Here's how the part is built. I have some questions about the finished solid (model axes, mm). A direction names the side the tool comes from. Give positions to 0.01 mm unless a question says otherwise; leave off trailing zeros. Loops run counter-clockwise (first coordinate to the right, second up) from the corner with the lowest first, then second, coordinate; pieces in that order, holes last.
Q1. I need wall thicknesses on probe 1 along X at (y, z) = (-7, 2.15) (3 decimals); probe 2 along Y at (x, z) = (52, 2.4) (3 decimals); probe 3 along X at (y, z) = (48, 2.1). Which ranges of each line are inside material? Lowest first, please.
Q2. Suppose I cut it at C-C (x = 69). List the corners of the cut face in (y, z) for me (3 decimals), and give its area (3 significant figures).
Q3. Thinking about a two-plate mould opening in X: for faces 1 (the face through (37, -4, 0)), 2 (the face through (28, -36.675, 1)), 3 (the face through (9, -17.625, 1)), 4 (the face through (-13.852, -62.211, 1.479)), which applies, pulls with the +X half, pulls with the -X half, needs draft (parallel to the pull), parting line crosses it, or undercut?
Q4. Suppose I cut it at D-D (z = 1.4). Count the separate pieces of the cut face and the enclosed holes in it, and give its area (3 significant figures).
Q5. Suppose I cut it at B-B (y = -1). List the corners of the cut face in (x, z) for me (3 decimals).
Q6. For faces 5 (the face through (28.817, 39, 1)), 6 (the face through (-15.278, -4, 1)), 7 (the face through (2.525, -44, 1)), which set-ups out of +Z, -Z, +X, -X, +Y, -Y let a thin tool reach every point of the face, with its end or its side?
Q7. I'm going to push flat-ended pins straight in: P1, Ø1, axis at x = 35, z = 1, coming from the +Y side; P2, Ø5, axis at x = 54, y = 35.5, coming from the -Z side. Where does each tip first touch, or does it pass through?
Q8. Suppose I cut it at A-A (y = 31). List the corners of the cut face in (x, z) for me, and give its area (3 significant figures).
```python
from build123d import *

# Parameters (mm, degrees)
SKETCH_R     = 1.7
PAD_DEPTH    = 3
POCKET_DEPTH = 10


with BuildPart() as part:
    # Sketch → Pad (new body)
    with BuildSketch(Plane.XY):
        with BuildLine():
            Line((-15.278, 48.916), (-15.278, -58.715))
            ThreePointArc((-15.278, -58.715), (-13.813534, -62.250534), (-10.278, -63.715))
            Line((-10.278, -63.715), (85.447, -63.715))
            ThreePointArc((85.447, -63.715), (88.982534, -62.250534), (90.447, -58.715))
            Line((90.447, -58.715), (90.447, 48.916))
            ThreePointArc((90.447, 48.916), (88.982534, 52.451534), (85.447, 53.916))
            Line((85.447, 53.916), (47.31676, 53.916))
            Line((47.31676, 22.916), (47.31676, 53.916))
            Line((28.81676, 22.916), (47.31676, 22.916))
            Line((28.81676, 53.916), (28.81676, 22.916))
            Line((28.81676, 53.916), (-10.278, 53.916))
            ThreePointArc((-10.278, 53.916), (-13.813534, 52.451534), (-15.278, 48.916))
        make_face()
        with Locations((-10.278, -58.715)):
            Circle(SKETCH_R, mode=Mode.SUBTRACT)
        with Locations((-10.278, 48.916)):
            Circle(SKETCH_R, mode=Mode.SUBTRACT)
        with Locations((85.447, 48.916)):
            Circle(SKETCH_R, mode=Mode.SUBTRACT)
        with Locations((85.447, -58.715)):
            Circle(SKETCH_R, mode=Mode.SUBTRACT)
    extrude(amount=PAD_DEPTH)

    # Sketch001 → Pocket (cut)
    with BuildSketch(Plane(origin=(0, 23, 0), x_dir=(1, 0, 0), z_dir=(0, 0, 1))):
        with BuildLine():
            ThreePointArc((73.175, -73.675), (73.528553, -73.528553), (73.675, -73.175))
            Line((73.675, -60.175), (73.675, -73.175))
            ThreePointArc((73.675, -60.175), (73.528553, -59.821447), (73.175, -59.675))
            Line((60.175, -59.675), (73.175, -59.675))
            ThreePointArc((60.175, -59.675), (59.821447, -59.821447), (59.675, -60.175))
            Line((59.675, -60.175), (59.675, -73.175))
            ThreePointArc((59.675, -73.175), (59.821447, -73.528553), (60.175, -73.675))
            Line((60.175, -73.675), (73.175, -73.675))
        make_face()
        with BuildLine():
            Line((3.025, -2.525), (16.025, -2.525))
            ThreePointArc((16.525, -3.025), (16.378553, -2.671447), (16.025, -2.525))
            Line((16.525, -3.025), (16.525, -16.025))
            ThreePointArc((16.025, -16.525), (16.378553, -16.378553), (16.525, -16.025))
            Line((3.025, -16.525), (16.025, -16.525))
            ThreePointArc((2.525, -16.025), (2.671447, -16.378553), (3.025, -16.525))
            Line((2.525, -3.025), (2.525, -16.025))
            ThreePointArc((3.025, -2.525), (2.671447, -2.671447), (2.525, -3.025))
        make_face()
        with BuildLine():
            Line((22.075, -2.525), (35.075, -2.525))
            ThreePointArc((35.575, -3.025), (35.428553, -2.671447), (35.075, -2.525))
            Line((35.575, -3.025), (35.575, -16.025))
            ThreePointArc((35.075, -16.525), (35.428553, -16.378553), (35.575, -16.025))
            Line((22.075, -16.525), (35.075, -16.525))
            ThreePointArc((21.575, -16.025), (21.721447, -16.378553), (22.075, -16.525))
            Line((21.575, -3.025), (21.575, -16.025))
            ThreePointArc((22.075, -2.525), (21.721447, -2.671447), (21.575, -3.025))
        make_face()
        with BuildLine():
            Line((41.125, -2.525), (54.125, -2.525))
            ThreePointArc((54.625, -3.025), (54.478553, -2.671447), (54.125, -2.525))
            Line((54.625, -3.025), (54.625, -16.025))
            ThreePointArc((54.125, -16.525), (54.478553, -16.378553), (54.625, -16.025))
            Line((41.125, -16.525), (54.125, -16.525))
            ThreePointArc((40.625, -16.025), (40.771447, -16.378553), (41.125, -16.525))
            Line((40.625, -3.025), (40.625, -16.025))
            ThreePointArc((41.125, -2.525), (40.771447, -2.671447), (40.625, -3.025))
        make_face()
        with BuildLine():
            Line((60.175, -2.525), (73.175, -2.525))
            ThreePointArc((73.675, -3.025), (73.528553, -2.671447), (73.175, -2.525))
            Line((73.675, -3.025), (73.675, -16.025))
            ThreePointArc((73.175, -16.525), (73.528553, -16.378553), (73.675, -16.025))
            Line((60.175, -16.525), (73.175, -16.525))
            ThreePointArc((59.675, -16.025), (59.821447, -16.378553), (60.175, -16.525))
            Line((59.675, -3.025), (59.675, -16.025))
            ThreePointArc((60.175, -2.525), (59.821447, -2.671447), (59.675, -3.025))
        make_face()
        with BuildLine():
            Line((3.025, -21.575), (16.025, -21.575))
            ThreePointArc((16.525, -22.075), (16.378553, -21.721447), (16.025, -21.575))
            Line((16.525, -22.075), (16.525, -35.075))
            ThreePointArc((16.025, -35.575), (16.378553, -35.428553), (16.525, -35.075))
            Line((3.025, -35.575), (16.025, -35.575))
            ThreePointArc((2.525, -35.075), (2.671447, -35.428553), (3.025, -35.575))
            Line((2.525, -22.075), (2.525, -35.075))
            ThreePointArc((3.025, -21.575), (2.671447, -21.721447), (2.525, -22.075))
        make_face()
        with BuildLine():
            Line((22.075, -21.575), (35.075, -21.575))
            ThreePointArc((35.575, -22.075), (35.428553, -21.721447), (35.075, -21.575))
            Line((35.575, -22.075), (35.575, -35.075))
            ThreePointArc((35.075, -35.575), (35.428553, -35.428553), (35.575, -35.075))
            Line((22.075, -35.575), (35.075, -35.575))
            ThreePointArc((21.575, -35.075), (21.721447, -35.428553), (22.075, -35.575))
            Line((21.575, -22.075), (21.575, -35.075))
            ThreePointArc((22.075, -21.575), (21.721447, -21.721447), (21.575, -22.075))
        make_face()
        with BuildLine():
            Line((41.125, -21.575), (54.125, -21.575))
            ThreePointArc((54.625, -22.075), (54.478553, -21.721447), (54.125, -21.575))
            Line((54.625, -22.075), (54.625, -35.075))
            ThreePointArc((54.125, -35.575), (54.478553, -35.428553), (54.625, -35.075))
            Line((41.125, -35.575), (54.125, -35.575))
            ThreePointArc((40.625, -35.075), (40.771447, -35.428553), (41.125, -35.575))
            Line((40.625, -22.075), (40.625, -35.075))
            ThreePointArc((41.125, -21.575), (40.771447, -21.721447), (40.625, -22.075))
        make_face()
        with BuildLine():
            Line((60.175, -21.575), (73.175, -21.575))
            ThreePointArc((73.675, -22.075), (73.528553, -21.721447), (73.175, -21.575))
            Line((73.675, -22.075), (73.675, -35.075))
            ThreePointArc((73.175, -35.575), (73.528553, -35.428553), (73.675, -35.075))
            Line((60.175, -35.575), (73.175, -35.575))
            ThreePointArc((59.675, -35.075), (59.821447, -35.428553), (60.175, -35.575))
            Line((59.675, -22.075), (59.675, -35.075))
            ThreePointArc((60.175, -21.575), (59.821447, -21.721447), (59.675, -22.075))
        make_face()
        with BuildLine():
            Line((3.025, -40.625), (16.025, -40.625))
            ThreePointArc((16.525, -41.125), (16.378553, -40.771447), (16.025, -40.625))
            Line((16.525, -41.125), (16.525, -54.125))
            ThreePointArc((16.025, -54.625), (16.378553, -54.478553), (16.525, -54.125))
            Line((3.025, -54.625), (16.025, -54.625))
            ThreePointArc((2.525, -54.125), (2.671447, -54.478553), (3.025, -54.625))
            Line((2.525, -41.125), (2.525, -54.125))
            ThreePointArc((3.025, -40.625), (2.671447, -40.771447), (2.525, -41.125))
        make_face()
        with BuildLine():
            Line((22.075, -40.625), (35.075, -40.625))
            ThreePointArc((35.575, -41.125), (35.428553, -40.771447), (35.075, -40.625))
            Line((35.575, -41.125), (35.575, -54.125))
            ThreePointArc((35.075, -54.625), (35.428553, -54.478553), (35.575, -54.125))
            Line((22.075, -54.625), (35.075, -54.625))
            ThreePointArc((21.575, -54.125), (21.721447, -54.478553), (22.075, -54.625))
            Line((21.575, -41.125), (21.575, -54.125))
            ThreePointArc((22.075, -40.625), (21.721447, -40.771447), (21.575, -41.125))
        make_face()
        with BuildLine():
            Line((41.125, -40.625), (54.125, -40.625))
            ThreePointArc((54.625, -41.125), (54.478553, -40.771447), (54.125, -40.625))
            Line((54.625, -41.125), (54.625, -54.125))
            ThreePointArc((54.125, -54.625), (54.478553, -54.478553), (54.625, -54.125))
            Line((41.125, -54.625), (54.125, -54.625))
            ThreePointArc((40.625, -54.125), (40.771447, -54.478553), (41.125, -54.625))
            Line((40.625, -41.125), (40.625, -54.125))
            ThreePointArc((41.125, -40.625), (40.771447, -40.771447), (40.625, -41.125))
        make_face()
        with BuildLine():
            Line((60.175, -40.625), (73.175, -40.625))
            ThreePointArc((73.675, -41.125), (73.528553, -40.771447), (73.175, -40.625))
            Line((73.675, -41.125), (73.675, -54.125))
            ThreePointArc((73.175, -54.625), (73.528553, -54.478553), (73.675, -54.125))
            Line((60.175, -54.625), (73.175, -54.625))
            ThreePointArc((59.675, -54.125), (59.821447, -54.478553), (60.175, -54.625))
            Line((59.675, -41.125), (59.675, -54.125))
            ThreePointArc((60.175, -40.625), (59.821447, -40.771447), (59.675, -41.125))
        make_face()
        with BuildLine():
            Line((3.025, -59.675), (16.025, -59.675))
            ThreePointArc((16.525, -60.175), (16.378553, -59.821447), (16.025, -59.675))
            Line((16.525, -60.175), (16.525, -73.175))
            ThreePointArc((16.025, -73.675), (16.378553, -73.528553), (16.525, -73.175))
            Line((3.025, -73.675), (16.025, -73.675))
            ThreePointArc((2.525, -73.175), (2.671447, -73.528553), (3.025, -73.675))
            Line((2.525, -60.175), (2.525, -73.175))
            ThreePointArc((3.025, -59.675), (2.671447, -59.821447), (2.525, -60.175))
        make_face()
        with BuildLine():
            Line((22.075, -59.675), (35.075, -59.675))
            ThreePointArc((35.575, -60.175), (35.428553, -59.821447), (35.075, -59.675))
            Line((35.575, -60.175), (35.575, -73.175))
            ThreePointArc((35.075, -73.675), (35.428553, -73.528553), (35.575, -73.175))
            Line((22.075, -73.675), (35.075, -73.675))
            ThreePointArc((21.575, -73.175), (21.721447, -73.528553), (22.075, -73.675))
            Line((21.575, -60.175), (21.575, -73.175))
            ThreePointArc((22.075, -59.675), (21.721447, -59.821447), (21.575, -60.175))
        make_face()
        with BuildLine():
            Line((41.125, -59.675), (54.125, -59.675))
            ThreePointArc((54.625, -60.175), (54.478553, -59.821447), (54.125, -59.675))
            Line((54.625, -60.175), (54.625, -73.175))
            ThreePointArc((54.125, -73.675), (54.478553, -73.528553), (54.625, -73.175))
            Line((41.125, -73.675), (54.125, -73.675))
            ThreePointArc((40.625, -73.175), (40.771447, -73.528553), (41.125, -73.675))
            Line((40.625, -60.175), (40.625, -73.175))
            ThreePointArc((41.125, -59.675), (40.771447, -59.821447), (40.625, -60.175))
        make_face()
    extrude(amount=POCKET_DEPTH, mode=Mode.SUBTRACT)


solid = part.part
```
Solutions:
1. probe 1: x = -15.278 to 2.525, 16.525 to 21.575, 35.575 to 40.625, 54.625 to 59.675, 73.675 to 90.447
1. probe 2: y = -63.715 to -50.675, -36.675 to -31.625, -17.625 to -12.575, 1.425 to 6.475, 20.475 to 53.916
1. probe 3: x = -15.28 to -11.71, -8.85 to 28.82, 47.32 to 84.01, 86.88 to 90.45
2. outline: (-63.715, 0) - (-50.675, 0) - (-50.675, 3) - (-63.715, 3) - close; (-36.675, 0) - (-31.625, 0) - (-31.625, 3) - (-36.675, 3) - close; (-17.625, 0) - (-12.575, 0) - (-12.575, 3) - (-17.625, 3) - close; (1.425, 0) - (6.475, 0) - (6.475, 3) - (1.425, 3) - close; (20.475, 0) - (53.916, 0) - (53.916, 3) - (20.475, 3) - close
2. area: 185 mm2
3. face 1: needs draft
3. face 2: undercut
3. face 3: undercut
3. face 4: pulls with the -X half
4. separate pieces: 1
4. enclosed holes: 20
4. area: 8,670 mm2
5. outline: (-15.278, 0) - (2.525, 0) - (2.525, 3) - (-15.278, 3) - close; (16.525, 0) - (21.575, 0) - (21.575, 3) - (16.525, 3) - close; (35.575, 0) - (40.625, 0) - (40.625, 3) - (35.575, 3) - close; (54.625, 0) - (59.675, 0) - (59.675, 3) - (54.625, 3) - close; (73.675, 0) - (90.447, 0) - (90.447, 3) - (73.675, 3) - close
6. face 5: +Z, -Z, +Y
6. face 6: +Z, -Z, -X, +Y, -Y
6. face 7: +Z, -Z
7. P1: stops at y = 22.92
7. P2: stops at z = 0
8. outline: (-15.28, 0) - (28.82, 0) - (28.82, 3) - (-15.28, 3) - close; (47.32, 0) - (90.45, 0) - (90.45, 3) - (47.32, 3) - close
8. area: 262 mm2
